```python
from build123d import *

# Parameters (mm, degrees)
SKETCH1_W           = 15.3
SKETCH1_H           = 5.8
BOSS_EXTRUDE1_DEPTH = 7
SKETCH3_W           = 13
SKETCH3_H           = 4.9
CUT_EXTRUDE1_DEPTH  = 5
SKETCH4_W           = 1.2
SKETCH4_H           = 3.5
CUT_EXTRUDE2_DEPTH  = 4
SKETCH5_W           = 15.3
SKETCH5_H           = 0.8
CUT_EXTRUDE3_DEPTH  = 0.8
SKETCH6_W           = 0.8
SKETCH6_H           = 0.8
CUT_EXTRUDE4_DEPTH  = 10
SKETCH7_W           = 13
SKETCH7_H           = 1
CUT_EXTRUDE5_DEPTH  = 0.3


with BuildPart() as part:
    # Sketch1 → Boss-Extrude1 (new body)
    with BuildSketch(Plane(origin=(0, 0, 0), x_dir=(1, 0, 0), z_dir=(0, 1, 0))):
        Rectangle(SKETCH1_W, SKETCH1_H)
    extrude(amount=BOSS_EXTRUDE1_DEPTH)

    # Sketch3 → Cut-Extrude1 (cut)
    with BuildSketch(Plane.XZ):
        Rectangle(SKETCH3_W, SKETCH3_H)
    extrude(amount=-CUT_EXTRUDE1_DEPTH, mode=Mode.SUBTRACT)

    # Sketch4 → Cut-Extrude2 (cut)
    with BuildSketch(Plane.XY.offset(2.9)):
        with Locations((-4.4, 1.75)):
            Rectangle(SKETCH4_W, SKETCH4_H)
        with Locations((4.4, 1.75)):
            Rectangle(SKETCH4_W, SKETCH4_H)
    extrude(amount=-CUT_EXTRUDE2_DEPTH, mode=Mode.SUBTRACT)

    # Sketch5 → Cut-Extrude3 (cut)
    with BuildSketch(Plane(origin=(0, 7, 0), x_dir=(1, 0, 0), z_dir=(0, 1, 0))):
        with Locations((0, 2.5)):
            Rectangle(SKETCH5_W, SKETCH5_H)
    extrude(amount=-CUT_EXTRUDE3_DEPTH, mode=Mode.SUBTRACT)

    # Sketch6 → Cut-Extrude4 (cut)
    with BuildSketch(Plane(origin=(0, 7, 0), x_dir=(1, 0, 0), z_dir=(0, 1, 0))):
        with Locations((4.8, -0.55)):
            Rectangle(SKETCH6_W, SKETCH6_H)
        with Locations((2.88, -0.55)):
            Rectangle(SKETCH6_W, SKETCH6_H)
        with Locations((0.96, -0.55)):
            Rectangle(SKETCH6_W, SKETCH6_H)
        with Locations((-0.96, -0.55)):
            Rectangle(SKETCH6_W, SKETCH6_H)
        with Locations((-2.88, -0.55)):
            Rectangle(SKETCH6_W, SKETCH6_H)
        with Locations((-4.8, -0.55)):
            Rectangle(SKETCH6_W, SKETCH6_H)
    extrude(amount=-CUT_EXTRUDE4_DEPTH, mode=Mode.SUBTRACT)

    # Sketch7 → Cut-Extrude5 (cut)
    with BuildSketch(Plane.XZ.offset(-5)):
        with Locations((0, -1.95)):
            Rectangle(SKETCH7_W, SKETCH7_H)
    extrude(amount=-CUT_EXTRUDE5_DEPTH, mode=Mode.SUBTRACT)


solid = part.part
```
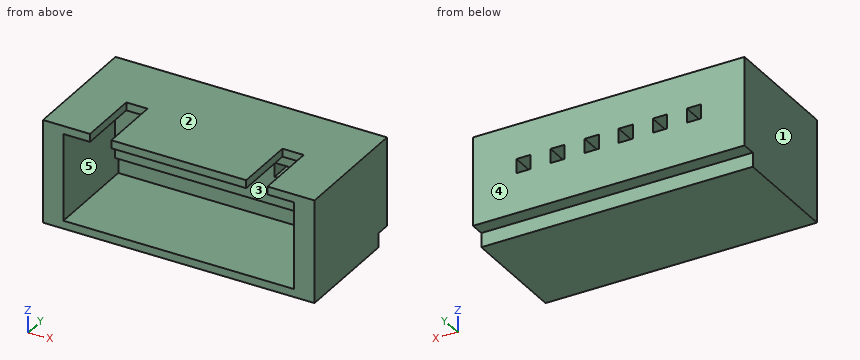
Geometry check sheet. Reference: the model listing, model coordinates, mm. Face numbers are marked on the shaded views. A direction names the side the tool comes from. Coordinates: 2 decimals unless noted, no trailing zeros. Order: outer loops, then holes, each group sorted by start corner. A loop starts at its lowest first (then second) coordinate and runs counter-clockwise, first axis right, second up.
Q1. Depth check by flat-ended pin: pin 1 Ø0.8 at (x, z) = (0, -2) entering from -Y. Enter the tip coordinate at first touch or a pass-through.
Reply:
pin 1: stops at y = 5.3
Q2. Sectioned sample at A-A on x = 0.75. Record the cut outline in (y, z).
Reply:
outline: (0, -2.9) - (6.2, -2.9) - (6.2, -2.1) - (7, -2.1) - (7, 0.15) - (5, 0.15) - (5, -1.45) - (5.3, -1.45) - (5.3, -2.45) - (0, -2.45) - close; (0, 2.45) - (5, 2.45) - (5, 0.95) - (7, 0.95) - (7, 2.9) - (0, 2.9) - close
Q3. Tool access check on the marked faces 4 and 5. Record the directions out of +Z, -Z, +X, -X, +Y, -Y that give a thin tool (end or side, any length) a straight path to the whole face; none if there is none.
Reply:
face 4: +Z, -Z, +X, -X, +Y
face 5: -Y
Q4. Sectioned sample at D-D on y = 4.25. Record the cut outline in (x, z).
Reply:
outline: (-7.65, -2.9) - (7.65, -2.9) - (7.65, 2.9) - (-7.65, 2.9) - close; hole (-6.5, -2.45) - (6.5, -2.45) - (6.5, 2.45) - (-6.5, 2.45) - close
Q5. Sectioned sample at C-C on z = 0.6. Give the number of separate pieces and of enclosed holes in the cut face, and give its area (3 significant figures).
Reply:
separate pieces: 7
enclosed holes: 0
area: 32.5 mm2
Q6. Sectioned sample at B-B on y = 3. Record the cut outline in (x, z), and give its area (3 significant figures).
Reply:
outline: (-7.65, -2.9) - (7.65, -2.9) - (7.65, 2.9) - (5, 2.9) - (5, 2.45) - (6.5, 2.45) - (6.5, -2.45) - (-6.5, -2.45) - (-6.5, 2.45) - (-5, 2.45) - (-5, 2.9) - (-7.65, 2.9) - close; (-3.8, 2.45) - (3.8, 2.45) - (3.8, 2.9) - (-3.8, 2.9) - close
area: 24.0 mm2
Q7. Draft check along X on the marked faces 1, 2 and 3. Enter one of: released by +X, released by -X, zero draft, split by the parting line, or undercut.
Reply:
face 1: released by -X
face 2: zero draft
face 3: undercut
Q8. Thickness scan on probe 1 along Z at (x, y) = (0, 2.25); probe 2 along X at (y, z) = (4, 1.25); probe 3 along Y at (x, z) = (-1.75, -1.8). Record the ranges inside material, lowest first.
Reply:
probe 1: z = -2.9 to -2.45, 2.45 to 2.9
probe 2: x = -7.65 to -6.5, 6.5 to 7.65
probe 3: y = 5.3 to 7
